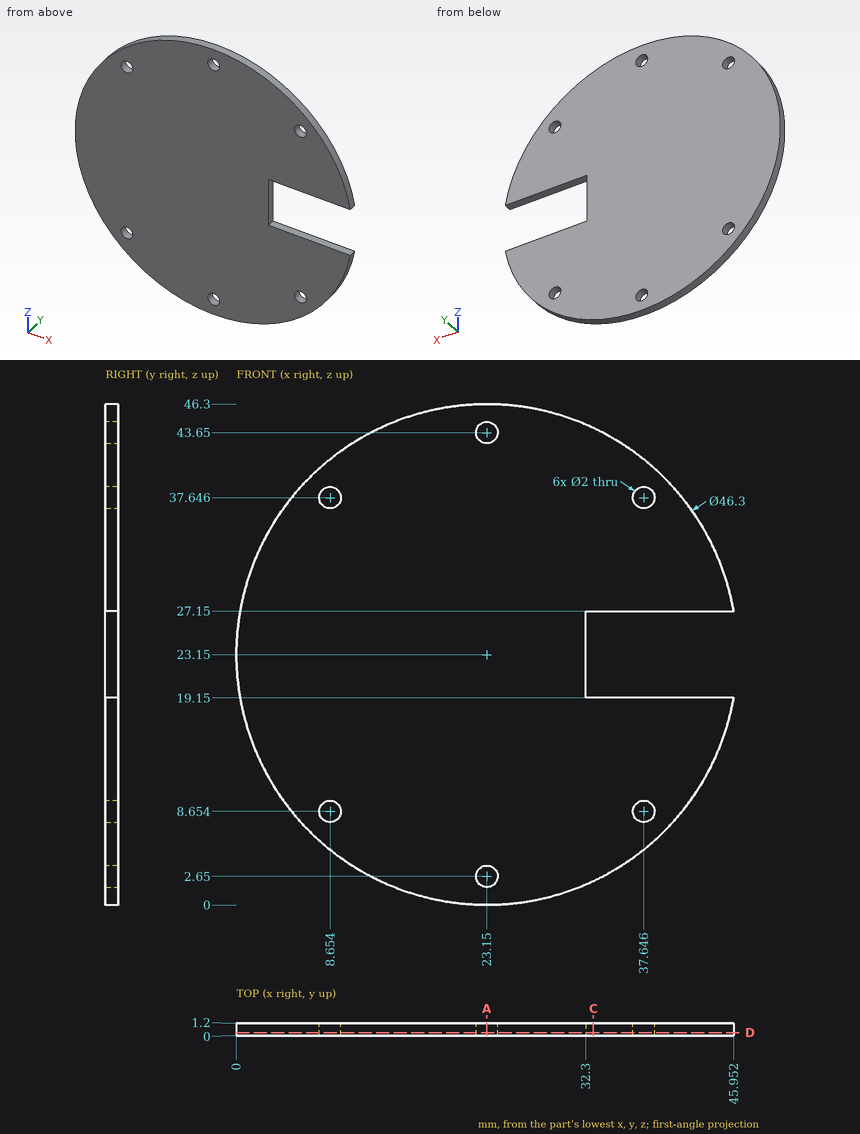
Answer from the drawing. Dimensions are ordinates in mm from the lowest x, y and z of the part. Coordinates: 2 decimals unless noted, no trailing zeros. Loops run counter-clockwise (first coordinate to the right, second up) from the corner with the lowest first, then second, coordinate; pieces in that order, holes last. Notation, with made-up numbers: (60.25, 1) -> (100.25, 1) arc R23 ccw to (100.25, 35) -> close; hole circle Ø11 at (35.5, 82.25). An arc over 180 degrees is marked (long way). Answer in a Markdown table with one row per item.
Item 1: Each of these flat-tipped pins is pushed along its axis until it touches: P1, Ø1.8, axis at x = 37.65, z = 8.65, coming from the -Y side; P2, Ø12, axis at x = 21, z = 24, coming from the -Y side; P3, Ø0.6, axis at y = 0.5, z = 23.5, coming from the +X side; P4, Ø0.6, axis at x = 42, y = 0.5, coming from the +Z side. Where does it stop, or does it pass through?
Returned:
| item | result |
|---|---|
| P1 | passes through |
| P2 | stops at y = 0 |
| P3 | stops at x = 32.3 |
| P4 | stops at z = 37 |
Item 2: A cutting plane is placed at C-C on x = 33. Determine the outline of the cut face in (y, z).
Returned:
| item | result |
|---|---|
| outline | (0, 2.2) -> (1.2, 2.2) -> (1.2, 19.15) -> (0, 19.15) -> close; (0, 27.15) -> (1.2, 27.15) -> (1.2, 44.1) -> (0, 44.1) -> close |
Item 3: Straight lines are drawn through the part: line 1 along Z through (x, y) = (24, 0.25) (1 decimal); line 2 along Z through (x, y) = (37, 0.15); line 3 along X through (y, z) = (1.05, 38). For each, find the intervals that lie inside material, in ascending order. Write a range as [from, to].
Returned:
| item | result |
|---|---|
| line 1 | z = [0, 2.1], [3.2, 43.1], [44.2, 46.3] |
| line 2 | z = [4.6, 7.89], [9.42, 19.15], [27.15, 36.88], [38.41, 41.7] |
| line 3 | x = [5.39, 7.72], [9.59, 36.71], [38.58, 40.91] |
Item 4: A cutting plane is placed at D-D on y = 0.3. Determine the outline of the cut face in (x, z).
Returned:
| item | result |
|---|---|
| outline | (32.3, 19.15) -> (32.3, 27.15) -> (45.95, 27.15) arc R23.15 ccw (long way) to (45.95, 19.15) -> close; hole circle Ø2 at (8.65, 8.65); hole circle Ø2 at (8.65, 37.65); hole circle Ø2 at (23.15, 2.65); hole circle Ø2 at (23.15, 43.65); hole circle Ø2 at (37.65, 8.65); hole circle Ø2 at (37.65, 37.65) |
Item 5: A cutting plane is placed at A-A on x = 23.15. Determine the outline of the cut face in (y, z).
Returned:
| item | result |
|---|---|
| outline | (0, 0) -> (1.2, 0) -> (1.2, 1.65) -> (0, 1.65) -> close; (0, 3.65) -> (1.2, 3.65) -> (1.2, 42.65) -> (0, 42.65) -> close; (0, 44.65) -> (1.2, 44.65) -> (1.2, 46.3) -> (0, 46.3) -> close |
